```python
from build123d import *

# Parameters (mm, degrees)
SKETCH1_R           = 1.5
BOSS_EXTRUDE1_DEPTH = 1.6129


with BuildPart() as part:
    # Sketch1 → Boss-Extrude1 (new body)
    with BuildSketch(Plane.XY):
        with BuildLine():
            Line((48.7, 32.8), (41.08, 32.8))
            Line((41.08, 32.8), (41.08, 45.5))
            Line((41.08, 45.5), (60.131959382, 45.5))
            ThreePointArc((60.131959382, 45.5), (75.061798197, -7.199235406), (50.387424414, -56.1))
            Line((50.387424414, -56.1), (-50.387424414, -56.1))
            ThreePointArc((-50.387424414, -56.1), (-75.061798197, -7.199235406), (-60.131959382, 45.5))
            Line((-60.131959382, 45.5), (-41.08, 45.5))
            Line((-41.08, 45.5), (-41.08, 32.8))
            Line((-41.08, 32.8), (-48.7, 32.8))
            Line((-48.7, 32.8), (-48.7, -7.4))
            Line((-48.7, -7.4), (48.7, -7.4))
            Line((48.7, -7.4), (48.7, 32.8))
        make_face()
        with Locations((-46.5, 40.199999991)):
            Circle(SKETCH1_R, mode=Mode.SUBTRACT)
        with Locations((46.5, 40.199999991)):
            Circle(SKETCH1_R, mode=Mode.SUBTRACT)
        with Locations((46.5, -14.799999991)):
            Circle(SKETCH1_R, mode=Mode.SUBTRACT)
        with Locations((-46.5, -14.799999991)):
            Circle(SKETCH1_R, mode=Mode.SUBTRACT)
    extrude(amount=BOSS_EXTRUDE1_DEPTH)


solid = part.part
```
The model under review builds one solid part; all positions refer to its coordinate system, in mm. Round coordinates to 2 decimals unless told otherwise and drop trailing zeros. Loops run counter-clockwise (first coordinate to the right, second up) from the corner with the lowest first, then second, coordinate; pieces in that order, holes last. Notation, with made-up numbers: M -19.75,13.25 L 32.25,13.25 A32 cw 32.25,42.25 Z; hole C 31,34.5 d6. An arc over 180 degrees is marked long. Write item = value, one per line.
Item 1: Take a section at B-B on z = 1.1. Write out the cut boundary in (x, y).
Return value:
outline = M -60.13,45.5 A75.41 ccw -50.39,-56.1 L 50.39,-56.1 A75.41 ccw 60.13,45.5 L 41.08,45.5 L 41.08,32.8 L 48.7,32.8 L 48.7,-7.4 L -48.7,-7.4 L -48.7,32.8 L -41.08,32.8 L -41.08,45.5 Z; hole C -46.5,-14.8 d3; hole C -46.5,40.2 d3; hole C 46.5,-14.8 d3; hole C 46.5,40.2 d3
Item 2: Take a section at C-C on y = 40.2. Write out the cut boundary in (x, z), then the cut area to 3 significant figures.
Return value:
outline = M -63.8,0 L -48,0 L -48,1.61 L -63.8,1.61 Z; M -45,0 L -41.08,0 L -41.08,1.61 L -45,1.61 Z; M 41.08,0 L 45,0 L 45,1.61 L 41.08,1.61 Z; M 48,0 L 63.8,0 L 63.8,1.61 L 48,1.61 Z
area = 63.6 mm2
Item 3: For line 1 (Y direction, x = 46.5, z = 1.2); line 2 (X direction, y = 40.2, z = 1.05); line 3 (Y direction, x = -16.5, z = 0.3), list the stretches that pass through material, from the lowest coordinate up. Write a range as [from, to].
Return value:
line_1 = [-56.1, -16.3], [-13.3, -7.4], [32.8, 38.7], [41.7, 45.5]
line_2 = [-63.8, -48], [-45, -41.08], [41.08, 45], [48, 63.8]
line_3 = [-56.1, -7.4]
Item 4: The part is to be moulded in two halves that separate along Y. For faces 1 (the cylindrical face through (-48, -14.73, 0.8)), 2 (the flat face through (1, -16, 1.613)), 3 (the cylindrical face through (-74.983, -7.98, 0.795)), say which applies: released by +Y, released by -Y, zero draft, split by the parting line, or undercut.
Return value:
face_1 = undercut
face_2 = zero draft
face_3 = split by the parting line
Item 5: Take a section at D-D on y = -14.8. Write out the cut boundary in (x, z), then the cut area to 3 significant figures.
Return value:
outline = M -73.94,0 L -48,0 L -48,1.61 L -73.94,1.61 Z; M -45,0 L 45,0 L 45,1.61 L -45,1.61 Z; M 48,0 L 73.94,0 L 73.94,1.61 L 48,1.61 Z
area = 229 mm2
Item 6: Insertion check: P1, Ø0.8, axis at y = 36.5, z = 1, coming from the +X side; P2, Ø1, axis at x = 51.5, y = -41, coming from the -Z side; P3, Ø0.8, axis at y = 19, z = 0.5, coming from the +X side; P4, Ø0.5, axis at y = 38.5, z = 1, coming from the -X side. Each pin has a flat end and moves straight along its axis. Give the tip position at first contact, or say it passes through.
Return value:
P1 = 66.2
P2 = 0
P3 = 73.08
P4 = -64.98
Item 7: Take a section at A-A on x = 46.5. Write out the cut boundary in (y, z).
Return value:
outline = M -56.1,0 L -16.3,0 L -16.3,1.61 L -56.1,1.61 Z; M -13.3,0 L -7.4,0 L -7.4,1.61 L -13.3,1.61 Z; M 32.8,0 L 38.7,0 L 38.7,1.61 L 32.8,1.61 Z; M 41.7,0 L 45.5,0 L 45.5,1.61 L 41.7,1.61 Z
